Solid Edge part; units mm, degrees
sketch "Sketch1" plane through (0, 0, 0) normal (0, 0, 1) x (1, 0, 0)
  line L0 (12.5, 7.5) -> (-12.5, 7.5)
  line L1 (-12.5, 7.5) -> (-12.5, -7.5)
  line L2 (-12.5, -7.5) -> (12.5, -7.5)
  line L3 (12.5, -7.5) -> (12.5, 7.5)
extrude "Protrusion1" add sketch "Sketch1" along normal blind 1
fillet "Round_1" radius 0.5 4 edges at (12.5, 7.5, 0.5) (12.5, -7.5, 0.5) (-12.5, -7.5, 0.5) (-12.5, 7.5, 0.5)
hole "Hole_1" at (-2.5, 0, 1) direction (0, 0, -1) diameter 3 end up to next
hole "Hole_2" at (-8, 5, 1) direction (0, 0, -1) diameter 1.5 end up to next
hole "Hole1" at (-8, 3, 1) direction (0, 0, -1) diameter 1.5 end up to next
hole "Hole2" at (-8, 1, 1) direction (0, 0, -1) diameter 1.5 end up to next
hole "Hole3" at (-8, -1, 1) direction (0, 0, -1) diameter 1.5 end up to next
hole "Hole4" at (-8, -3, 1) direction (0, 0, -1) diameter 1.5 end up to next
hole "Hole5" at (-8, -5, 1) direction (0, 0, -1) diameter 1.5 end up to next
Part model, mm, in its own coordinate system. Give positions to 0.01 mm unless a question says otherwise; leave off trailing zeros. Loops run counter-clockwise (first coordinate to the right, second up) from the corner with the lowest first, then second, coordinate; pieces in that order, holes last. Notation, with made-up numbers: M 33.25,67.25 L 46.25,67.25 A9 ccw 46.25,74.25 Z; hole C 63,27 d8. An arc over 180 degrees is marked long. Return JSON: item names as keys, results as strings.
1) Pull direction Y, two halves, no side cores. Call faces 1 (the face through (12.5, -0.1, 0.5)), 2 (the face through (-7.97, 5.75, 0.51)), 3 (the face through (0.2, 7.5, 0.5)): released by +Y, released by -Y, zero draft, split by the parting line, or undercut.
Calculated:
{"face 1": "zero draft", "face 2": "undercut", "face 3": "released by +Y"}
2) Saw through at C-C, the plane y = -5. List the corners of the cut face in (x, z).
Calculated:
{"outline": "M -12.5,0 L -8.75,0 L -8.75,1 L -12.5,1 Z; M -7.25,0 L 12.5,0 L 12.5,1 L -7.25,1 Z"}
3) Drill centre lines: line 1 (X direction, y = 0, z = 0.6); line 2 (X direction, y = -1, z = 0.2); line 3 (X direction, y = 5, z = 0.85). Where is each one in solid material? Low to high.
Calculated:
{"line 1": "x = -12.5 to -4, -1 to 12.5", "line 2": "x = -12.5 to -8.75, -7.25 to -3.62, -1.38 to 12.5", "line 3": "x = -12.5 to -8.75, -7.25 to 12.5"}
4) Saw through at A-A, the plane y = 0. List the corners of the cut face in (x, z), then the cut area to 3 significant figures.
Calculated:
{"outline": "M -12.5,0 L -4,0 L -4,1 L -12.5,1 Z; M -1,0 L 12.5,0 L 12.5,1 L -1,1 Z", "area": "22.0 mm2"}
5) Flat gauge pin, fed straight in: pin 1 Ø1.7 at (x, y) = (-8, -1) entering from +Z. Where does the tip first touch, or does it go through?
Calculated:
{"pin 1": "stops at z = 1"}
6) Saw through at B-B, the plane z = 0.6. List the corners of the cut face in (x, y), then the cut area to 3 significant figures.
Calculated:
{"outline": "M -12.5,-7 A0.5 ccw -12,-7.5 L 12,-7.5 A0.5 ccw 12.5,-7 L 12.5,7 A0.5 ccw 12,7.5 L -12,7.5 A0.5 ccw -12.5,7 Z; hole C -8,-5 d1.5; hole C -8,-3 d1.5; hole C -8,-1 d1.5; hole C -8,1 d1.5; hole C -8,3 d1.5; hole C -8,5 d1.5; hole C -2.5,0 d3", "area": "357 mm2"}
